```python
from build123d import *

# Parameters (mm, degrees)
F2_DEPTH = 50.8
F5_DEPTH = 50.8
F5_TAPER = 40


with BuildPart() as f2:
    # F1 (on Top) → F2 (new body)
    with BuildSketch(Plane.XY):
        Polygon((71.0278424351, -0.688096386), (36.109830168, 61.1678677318), (-34.9180122671, 61.8559641178), (-71.0278424351, 0.688096386), (-36.109830168, -61.1678677318), (34.9180122671, -61.8559641178), align=None)
    extrude(amount=-F2_DEPTH)

    # F3 (on offset) → F4 section 0
    with BuildSketch(Plane.XY.offset(38.1)):
        Polygon((6.3483007252, -10.7696512714), (12.5009419535, 0.1129640632), (6.1526412283, 10.8826153346), (-6.3483007252, 10.7696512714), (-12.5009419535, -0.1129640632), (-6.1526412283, -10.8826153346), align=None)
    # F2_face (on face) → F4 section 1
    with BuildSketch(Plane.XY):
        Polygon((71.0278424351, -0.688096386), (36.109830168, 61.1678677318), (-34.9180122671, 61.8559641178), (-71.0278424351, 0.688096386), (-36.109830168, -61.1678677318), (34.9180122671, -61.8559641178), align=None)
    loft()

    # F4_face (on face) → F5 (join)
    with BuildSketch(Plane.XY.offset(38.1)):
        Polygon((-6.1526412283, -10.8826153346), (6.3483007252, -10.7696512714), (12.5009419535, 0.1129640632), (6.1526412283, 10.8826153346), (-6.3483007252, 10.7696512714), (-12.5009419535, -0.1129640632), align=None)
    extrude(amount=F5_DEPTH, taper=F5_TAPER)


solid = f2.part
```
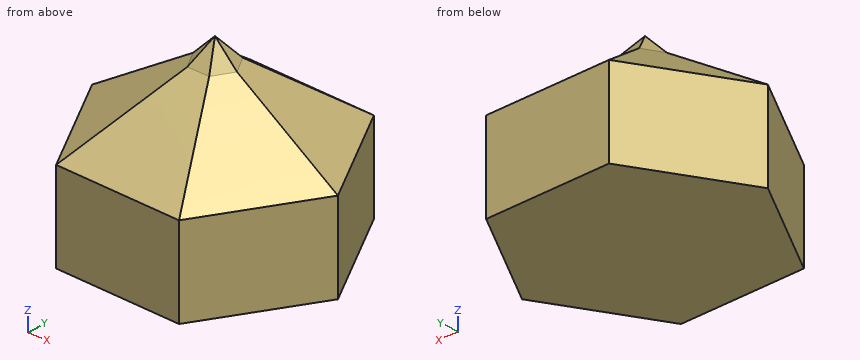
Here's how the part is built. I have some questions about the finished solid (model axes, mm). Round coordinates to 2 decimals unless told otherwise and drop trailing zeros. Write each loop counter-clockwise with the first axis right and the second up, starting at its lowest first coordinate (ties: lowest second). Pieces come first, ordered by that corner, then holes. Notation, with made-up numbers: M 26.5,-3 L 76.5,-3 A16 ccw 76.5,27 Z; hole C 19.25,82 d9. An arc over 180 degrees is marked long. Answer as CSV lines item,"result". Start each with the question number.
1. I need wall thicknesses on probe 1 along Z at (x, y) = (-14, 16); probe 2 along Y at (x, z) = (-19.5, 10); probe 3 along Z at (x, y) = (-1, 16.5). Which ranges of each line are inside material? Lowest first, please.
2. Suppose I cut it at B-B on z = 44. Write out the boundary of the cut face in (x, y) (3 decimals), then the cut area to 3 significant figures.
3. Suppose I cut it at A-A on z = -20.5. Write out the boundary of the cut face in (x, y), then the cut area to 3 significant figures.
4. I'm going to push flat-ended pins straight in: pin 1 Ø4 at (y, z) = (39, 14.5) entering from -X; pin 2 Ø5 at (x, y) = (-6, 23.5) entering from +Z; pin 3 Ø5 at (x, z) = (28, -1.5) entering from +Y. Where does each tip first touch, or does it pass through?
Check result:
1,probe 1,"z = -50.8 to 31.1"
1,probe 2,"y = -48.04 to 48.38"
1,probe 3,"z = -50.8 to 33.83"
2,outline,"M -6.785,-0.061 L -3.339,-5.906 L 3.445,-5.845 L 6.785,0.061 L 3.339,5.906 L -3.445,5.845 Z"
2,area,"120 mm2"
3,outline,"M -71.03,0.69 L -36.11,-61.17 L 34.92,-61.86 L 71.03,-0.69 L 36.11,61.17 L -34.92,61.86 Z"
3,area,"13,100 mm2"
4,pin 1,"stops at x = -29.35"
4,pin 2,"stops at z = 30.46"
4,pin 3,"stops at y = 61.27"
